Check sheet for the drawn part. Datum: minimum x, y, z corner. Units: mm. Round coordinates to 2 decimals unless told otherwise and drop trailing zeros. Write each loop counter-clockwise with the first axis right and the second up, starting at its lowest first coordinate (ties: lowest second). Pieces come first, ordered by that corner, then holes. Notation, with made-up numbers: (50, 14) - (68, 14) arc R14 cw to (68, 21) - close; hole circle Ø3 at (78, 71). An arc over 180 degrees is marked (long way). Write each question's results on one line, items separated by ' | '.
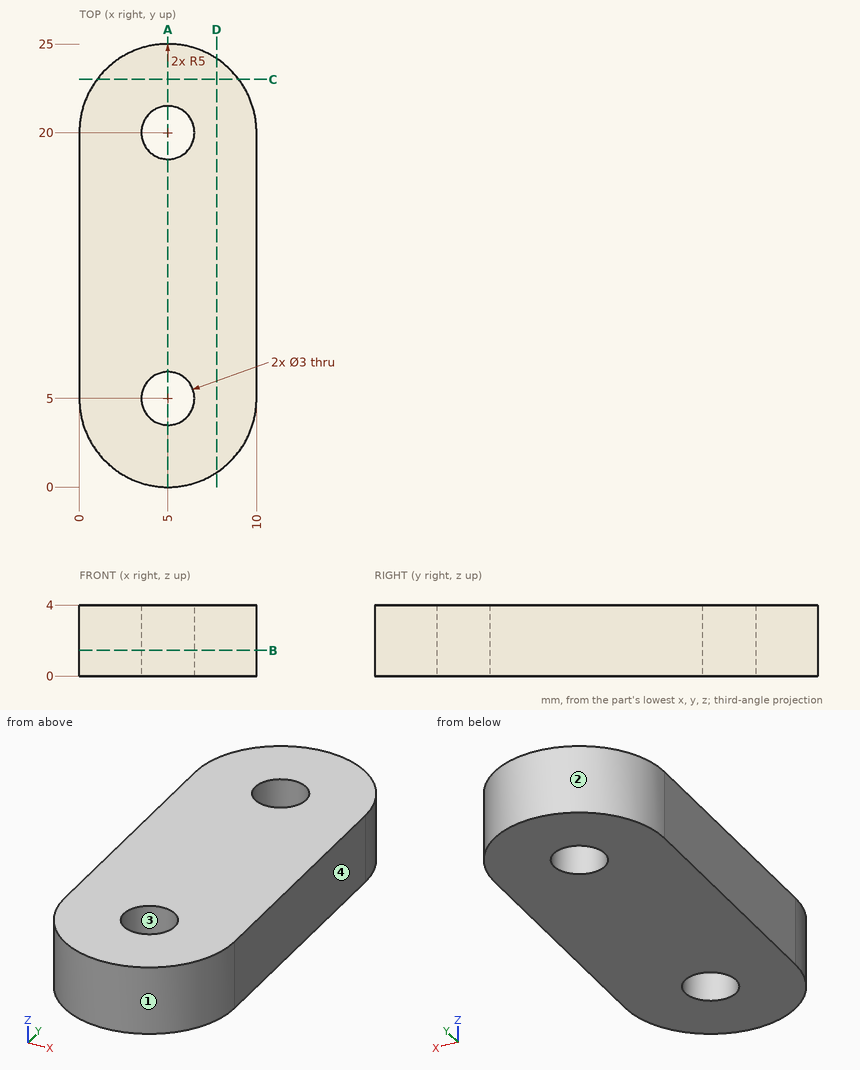
(1) Thickness scan on L1, parallel to Y at x = 5, z = 2.85; L2, parallel to Y at x = 4.25, z = 1.4; L3, parallel to X at y = 21.75, z = 3.4. Record the ranges inside material, lowest first.
Answer:
L1: 0 to 3.5, 6.5 to 18.5, 21.5 to 25 | L2: 0.06 to 3.7, 6.3 to 18.7, 21.3 to 24.94 | L3: 0.32 to 9.68
(2) Section check D-D (x = 7.75). Record the cut outline in (y, z).
Answer:
outline: (0.82, 0) - (24.18, 0) - (24.18, 4) - (0.82, 4) - close
(3) Section check B-B (z = 1.45). Record the cut outline in (x, y).
Answer:
outline: (0, 5) arc R5 ccw to (10, 5) - (10, 20) arc R5 ccw to (0, 20) - close; hole circle Ø3 at (5, 5); hole circle Ø3 at (5, 20)
(4) Section check A-A (x = 5). Record the cut outline in (y, z).
Answer:
outline: (0, 0) - (3.5, 0) - (3.5, 4) - (0, 4) - close; (6.5, 0) - (18.5, 0) - (18.5, 4) - (6.5, 4) - close; (21.5, 0) - (25, 0) - (25, 4) - (21.5, 4) - close
(5) Go/stop test with flat-tipped pins: pin 1 Ø2.5 at (x, y) = (5, 20) entering from +Z; pin 2 Ø1 at (x, z) = (8.5, 3.5) entering from -Y. Record where each tip stops, or that it passes through.
Answer:
pin 1: through | pin 2: y = 1
(6) Section check C-C (y = 23). Record the cut outline in (x, z).
Answer:
outline: (1, 0) - (9, 0) - (9, 4) - (1, 4) - close
(7) Mould release check, pull along Y, two halves, no side actions. Record for the marked faces 1, 2, 3 and 4: released by +Y, released by -Y, zero draft, split by the parting line, or undercut.
Answer:
face 1: released by -Y | face 2: released by +Y | face 3: undercut | face 4: zero draft
